```python
from build123d import *

# Parameters (mm, degrees)
SKETCH1_W               = 25.4
SKETCH1_H               = 25.4
SKETCH1_W_2             = 19.05
SKETCH1_H_2             = 19.05
EXTRUDE_THIN1_DEPTH     = 711.2
F_10_CLEARANCE_HOLE1_D  = 5.1054
LPATTERN1_COUNT         = 11
LPATTERN1_PITCH         = 63.5
F_10_CLEARANCE_HOLE2_D  = 5.1054
F_10_CLEARANCE_HOLE3_D  = 5.1054
CUT_EXTRUDE1_DEPTH      = 713.106565059
CUT_EXTRUDE1_DEPTH_BACK = 713.106565059
SKETCH8_R               = 9.525


with BuildPart() as part:
    # Sketch1 → Extrude-Thin1 (new body)
    with BuildSketch(Plane.XY):
        with Locations((-12.7, 12.7)):
            Rectangle(SKETCH1_W, SKETCH1_H)
        with Locations((-12.7, 12.7)):
            Rectangle(SKETCH1_W_2, SKETCH1_H_2, mode=Mode.SUBTRACT)
    extrude(amount=EXTRUDE_THIN1_DEPTH)

    # #10 Clearance Hole1 (through all)
    with Locations(Plane(origin=(0, 25.4, 0), x_dir=(1, 0, 0), z_dir=(0, 1, 0))):
        with Locations((-12.7, -673.1)):
            f_10_clearance_hole1 = Hole(F_10_CLEARANCE_HOLE1_D / 2)

    # LPattern1: #10 Clearance Hole1 ×11
    with Locations(*[(0, 0, -i * LPATTERN1_PITCH) for i in range(1, LPATTERN1_COUNT)]):
        add(f_10_clearance_hole1, mode=Mode.SUBTRACT)

    # #10 Clearance Hole2 (through all)
    with Locations(Plane(origin=(0, 0, 0), x_dir=(0, 0, -1), z_dir=(1, 0, 0))):
        with Locations((-698.5, 12.7), (-685.8, 12.7), (-673.1, 12.7)):
            Hole(F_10_CLEARANCE_HOLE2_D / 2)

    # #10 Clearance Hole3 (through all)
    with Locations(Plane(origin=(0, 0, 0), x_dir=(0, 0, -1), z_dir=(1, 0, 0))):
        with Locations((-38.1, 12.7), (-25.4, 12.7), (-12.7, 12.7)):
            Hole(F_10_CLEARANCE_HOLE3_D / 2)

    # Sketch8 → Cut-Extrude1 (cut, two sides: drawn at the far end of the back side and taken through both)
    with BuildSketch(Plane.ZY.offset(25.4).offset(-CUT_EXTRUDE1_DEPTH_BACK)):
        with Locations(Location((330.2, 12.7, 0), (0, 0, 270))):
            Circle(SKETCH8_R)
    extrude(amount=CUT_EXTRUDE1_DEPTH + CUT_EXTRUDE1_DEPTH_BACK, mode=Mode.SUBTRACT)


solid = part.part
```
Geometry: final body of the model. Coordinates: model frame, mm. A direction names the side the tool comes from. Round coordinates to 2 decimals unless told otherwise and drop trailing zeros. Write each loop counter-clockwise with the first axis right and the second up, starting at its lowest first coordinate (ties: lowest second). Pieces come first, ordered by that corner, then holes.
Item 1: Section query A-A (z = 114). Return loops of the section in (x, y) (3 decimals).
Item 2: Mould query, pull axis Y, two halves, no side actions, for faces 1 (the face through (-2, 13, 711.2)), 2 (the face through (-13, 25.4, 351)), 3 (the face through (-22.225, 13, 163)). Classes: +Y half, -Y half, draft (parallel to the pull), parting line (faces both ways), or undercut.
Item 3: Pin query (flat end, axial travel): P1, Ø3, axis at x = -12.7, z = 292.1, coming from the -Y side. Return the tip coordinate at first contact, or that it passes through.
Item 4: Set-up query: faces 4 (the face through (-25.4, 13, 351)), 5 (the face through (-3.175, 13, 163)). Return all of +Z, -Z, +X, -X, +Y, -Y with unobstructed straight access to the full face (end or side cutting, diameter ignored); none if empty.
Item 5: Material intervals for L1, parallel to Y at x = -14.25, z = 62.5 (3 decimals); L2, parallel to X at y = 5, z = 121 (3 decimals); L3, parallel to X at y = 2, z = 609.6, sorted ascending.
Completed:
1. outline: (-25.4, 0) - (0, 0) - (0, 25.4) - (-25.4, 25.4) - close; hole (-22.225, 3.175) - (-3.175, 3.175) - (-3.175, 22.225) - (-22.225, 22.225) - close
2. face 1: draft
2. face 2: +Y half
2. face 3: undercut
3. P1: passes through
4. face 4: +Z, -Z, -X, +Y, -Y
4. face 5: +Z, -Z
5. L1: y = 0 to 3.175, 22.225 to 25.4
5. L2: x = -25.4 to -22.225, -3.175 to 0
5. L3: x = -25.4 to -15.25, -10.15 to 0
